Geometry: final body of the model. Coordinates: model frame, mm. A direction names the side the tool comes from. Give positions to 0.01 mm unless a question says otherwise; leave off trailing zeros. Write each loop counter-clockwise with the first axis right and the second up, starting at its lowest first coordinate (ties: lowest second). Pieces come first, ordered by that corner, then holes. Notation, with made-up numbers: M -25,40 L 9,40 A34 cw 9,72 Z; hole C -21.75,25.5 d5. An arc over 180 degrees is marked long. Use a Markdown table: item, result. Add a question column.
1) Section A-A on y = -76.5. Return the cut outline in (x, z).
2) Section B-B on y = -161.5. Return the cut outline in (x, z), then the cut area to 3 significant figures.
3) Pin query (flat end, axial travel): pin 1 (5 mm diameter, centred on x = -15, y = -105.5, fed in from +Z); pin 2 (1.9 mm diameter, centred on y = -106.5, z = -16, fed in from +X); pin 3 (8 mm diameter, centred on x = -1, y = -110.5, fed in from -Z). Return the tip coordinate at first contact, or that it passes through.
4) Set-up query: faces 1 (the flat face through (35.387, -109, -16)), 2 (the flat face through (-23.069, -109, 5)), 3 (the cylindrical face through (-10.214, -149.991, -7.832)). Return all of +Z, -Z, +X, -X, +Y, -Y with unobstructed straight access to the full face (end or side cutting, diameter ignored); none if empty.
5) Line query: line 1 (Y direction, x = 29.5, z = -5); line 2 (Z direction, x = -11.5, y = -71.5); line 3 (X direction, y = -71, z = 17). Output: solid intervals per line, ascending.
```python
from build123d import *

# Parameters (mm, degrees)
F0_W     = 78.0319198966
F0_H     = 74.7814178467
F1_DEPTH = 95.6868380308
F2_R     = 58.5481836396
F3_R     = 14.8908027662
F4_R     = 9.7880573939
F5_R     = 12.9631428279
F6_DEPTH = 31.8753421307
F7_SIZE  = 5.08
F8_R     = 12.871399231
F9_DEPTH = 53.6622554064
F10_R    = 8.1683236061


with BuildPart() as f1:
    # F0 (on Front) → F1 (new body)
    with BuildSketch(Plane.XZ):
        with Locations((6.1589442194, 8.3135068417)):
            Rectangle(F0_W, F0_H)
    extrude(amount=F1_DEPTH)

    # F2
    f2_edges = [f1.edges().sort_by_distance(p)[0] for p in [
        (45.174904, -47.843419, 45.704216),
    ]]
    fillet(f2_edges, radius=F2_R)

    # F3
    f3_edges = [f1.edges().sort_by_distance(p)[0] for p in [
        (-32.857016, -47.843419, 45.704216),
    ]]
    fillet(f3_edges, radius=F3_R)

    # F4
    f4_edges = [f1.edges().sort_by_distance(p)[0] for p in [
        (-15.669746, -95.686838, 45.704216),
        (-28.495601, -95.686838, 41.342801),
        (28.026538, -95.686838, 28.55585),
        (-32.857016, -95.686838, 0.868105),
        (45.174904, -95.686838, -20.960585),
        (6.158944, -95.686838, -29.077202),
    ]]
    fillet(f4_edges, radius=F4_R)

    # F5
    f5_edges = [f1.edges().sort_by_distance(p)[0] for p in [
        (28.026538, 0, 28.55585),
        (-15.669746, 0, 45.704216),
        (-28.495601, 0, 41.342801),
        (-32.857016, 0, 0.868105),
        (45.174904, 0, -20.960585),
        (6.158944, 0, -29.077202),
    ]]
    fillet(f5_edges, radius=F5_R)

    # F6 (add): a face of the model
    f6_faces = [f1.faces().sort_by_distance(p)[0] for p in [
        (2.7661274156, -95.6868380308, 5.1141155416),
    ]]
    extrude(f6_faces, amount=F6_DEPTH)

    # F7
    f7_edges = [f1.edges().sort_by_distance(p)[0] for p in [
        (35.386847, -127.56218, -16.066556),
        (6.158944, -127.56218, -19.289145),
        (21.105336, -127.56218, 21.634648),
        (-23.068958, -127.56218, 5.762134),
        (-15.669746, -127.56218, 35.916158),
        (-21.574399, -127.56218, 34.421599),
    ]]
    chamfer(f7_edges, length=F7_SIZE)

    # F8 (on face) → F9 (join)
    with BuildSketch(Plane.XZ.offset(127.5621801615)):
        Circle(F8_R)
    extrude(amount=F9_DEPTH)

    # F10
    f10_edges = [f1.edges().sort_by_distance(p)[0] for p in [
        (-12.871399, -181.224436, 0),
    ]]
    fillet(f10_edges, radius=F10_R)


solid = f1.part
```
Found:
| question | item | result |
|---|---|---|
| 1 | outline | M -32.86,-29.08 L 45.17,-29.08 L 45.17,-12.84 A58.55 ccw -13.37,45.7 L -17.97,45.7 A14.89 ccw -32.86,30.81 Z |
| 2 | outline | C 0,0 d25.74 |
| 2 | area | 520 mm² |
| 3 | pin 1 | z = 35.92 |
| 3 | pin 2 | x = 35.39 |
| 3 | pin 3 | z = -19.29 |
| 4 | face 1 | +Z, -Z, +X, -Y |
| 4 | face 2 | +Z, -Z, -X, -Y |
| 4 | face 3 | -Y |
| 5 | line 1 | -127.56 to 0 |
| 5 | line 2 | -29.08 to 45.67 |
| 5 | line 3 | -32.86 to 37 |
